Here's how the part is built. I have some questions about the finished solid (model axes, mm). Give positions to 0.01 mm unless a question says otherwise; leave off trailing zeros. Order: outer loops, then holes, each group sorted by start corner. A loop starts at its lowest first (then second) coordinate and runs counter-clockwise, first axis right, second up.
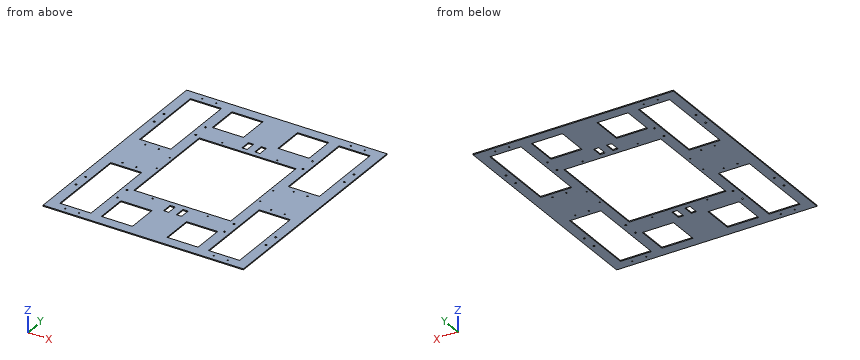
from build123d import *

# Parameters (mm, degrees)
SKETCH_1_W          = 580
SKETCH_1_H          = 660
EXTRUDE_1_DEPTH     = 3
SKETCH_2_W          = 90
SKETCH_2_H          = 233.23
CUT_EXTRUDE_1_DEPTH = 3
SKETCH_3_W          = 90
SKETCH_3_H          = 90
CUT_EXTRUDE_2_DEPTH = 4
SKETCH_4_W          = 280
SKETCH_4_H          = 300
CUT_EXTRUDE_3_DEPTH = 3
SKETCH_5_W          = 15
SKETCH_5_H          = 30
CUT_EXTRUDE_4_DEPTH = 3
SKETCH_6_R          = 2
CUT_EXTRUDE_5_DEPTH = 4
SKETCH_7_R          = 2.75
CUT_EXTRUDE_6_DEPTH = 4
SKETCH_8_R          = 2
CUT_EXTRUDE_7_DEPTH = 3


with BuildPart() as part:
    # 草圖1 → 填料-伸長1 (new body)
    with BuildSketch(Plane.XY):
        with Locations((-114.793886735, -166.775956284)):
            Rectangle(SKETCH_1_W, SKETCH_1_H)
    extrude(amount=EXTRUDE_1_DEPTH)

    # 草圖2 → 除料-伸長1 (cut)
    with BuildSketch(Plane.XY.offset(3)):
        with Locations((-329.793886735, -350.160956284)):
            Rectangle(SKETCH_2_W, SKETCH_2_H)
        with Locations((100.206113265, -350.160956284)):
            Rectangle(SKETCH_2_W, SKETCH_2_H)
        with Locations((100.206113265, 16.609043716)):
            Rectangle(SKETCH_2_W, SKETCH_2_H)
        with Locations((-329.793886735, 16.609043716)):
            Rectangle(SKETCH_2_W, SKETCH_2_H)
    extrude(amount=-CUT_EXTRUDE_1_DEPTH, mode=Mode.SUBTRACT)

    # 草圖3 → 除料-伸長2 (cut, through all)
    with BuildSketch(Plane.XY.offset(3)):
        with Locations((-209.793886735, -421.775956284)):
            Rectangle(SKETCH_3_W, SKETCH_3_H)
        with Locations((-19.793886735, -421.775956284)):
            Rectangle(SKETCH_3_W, SKETCH_3_H)
        with Locations((-19.793886735, 88.224043716)):
            Rectangle(SKETCH_3_W, SKETCH_3_H)
        with Locations((-209.793886735, 88.224043716)):
            Rectangle(SKETCH_3_W, SKETCH_3_H)
    extrude(amount=-CUT_EXTRUDE_2_DEPTH, mode=Mode.SUBTRACT)

    # 草圖4 → 除料-伸長3 (cut)
    with BuildSketch(Plane.XY.offset(3)):
        with Locations((-114.793886735, -166.775956284)):
            Rectangle(SKETCH_4_W, SKETCH_4_H)
    extrude(amount=-CUT_EXTRUDE_3_DEPTH, mode=Mode.SUBTRACT)

    # 草圖5 → 除料-伸長4 (cut)
    with BuildSketch(Plane.XY.offset(3)):
        with Locations((-96.293886735, -346.775956284)):
            Rectangle(SKETCH_5_W, SKETCH_5_H)
        with Locations((-133.293886735, -346.775956284)):
            Rectangle(SKETCH_5_W, SKETCH_5_H)
        with Locations((-133.293886735, 13.224043716)):
            Rectangle(SKETCH_5_W, SKETCH_5_H)
        with Locations((-96.293886735, 13.224043716)):
            Rectangle(SKETCH_5_W, SKETCH_5_H)
    extrude(amount=-CUT_EXTRUDE_4_DEPTH, mode=Mode.SUBTRACT)

    # 草圖6 → 除料-伸長5 (cut, through all)
    with BuildSketch(Plane.XY.offset(3)):
        with Locations((-349.793886735, -218.545956284)):
            Circle(SKETCH_6_R)
        with Locations((-309.793886735, -218.545956284)):
            Circle(SKETCH_6_R)
        with Locations((-309.793886735, -481.775956284)):
            Circle(SKETCH_6_R)
        with Locations((-349.793886735, -481.775956284)):
            Circle(SKETCH_6_R)
        with Locations((80.206113265, -481.775956284)):
            Circle(SKETCH_6_R)
        with Locations((120.206113265, -481.775956284)):
            Circle(SKETCH_6_R)
        with Locations((80.206113265, -218.545956284)):
            Circle(SKETCH_6_R)
        with Locations((120.206113265, -218.545956284)):
            Circle(SKETCH_6_R)
        with Locations((-309.793886735, 148.224043716)):
            Circle(SKETCH_6_R)
        with Locations((-349.793886735, 148.224043716)):
            Circle(SKETCH_6_R)
        with Locations((-309.793886735, -115.005956284)):
            Circle(SKETCH_6_R)
        with Locations((-349.793886735, -115.005956284)):
            Circle(SKETCH_6_R)
        with Locations((80.206113265, -115.005956284)):
            Circle(SKETCH_6_R)
        with Locations((120.206113265, -115.005956284)):
            Circle(SKETCH_6_R)
        with Locations((120.206113265, 148.224043716)):
            Circle(SKETCH_6_R)
        with Locations((80.206113265, 148.224043716)):
            Circle(SKETCH_6_R)
    extrude(amount=-CUT_EXTRUDE_5_DEPTH, mode=Mode.SUBTRACT)

    # 草圖7 → 除料-伸長6 (cut, through all)
    with BuildSketch(Plane.XY.offset(3)):
        with Locations((-389.793886735, -368.775956284)):
            Circle(SKETCH_7_R)
        with Locations((-389.793886735, -324.775956284)):
            Circle(SKETCH_7_R)
        with Locations((-269.793886735, -324.775956284)):
            Circle(SKETCH_7_R)
        with Locations((-269.793886735, -368.775956284)):
            Circle(SKETCH_7_R)
        with Locations((40.206113265, -368.775956284)):
            Circle(SKETCH_7_R)
        with Locations((40.206113265, -324.775956284)):
            Circle(SKETCH_7_R)
        with Locations((160.206113265, -324.775956284)):
            Circle(SKETCH_7_R)
        with Locations((160.206113265, -368.775956284)):
            Circle(SKETCH_7_R)
        with Locations((160.206113265, 35.224043716)):
            Circle(SKETCH_7_R)
        with Locations((160.206113265, -8.775956284)):
            Circle(SKETCH_7_R)
        with Locations((40.206113265, -8.775956284)):
            Circle(SKETCH_7_R)
        with Locations((40.206113265, 35.224043716)):
            Circle(SKETCH_7_R)
        with Locations((-269.793886735, 35.224043716)):
            Circle(SKETCH_7_R)
        with Locations((-269.793886735, -8.775956284)):
            Circle(SKETCH_7_R)
        with Locations((-389.793886735, -8.775956284)):
            Circle(SKETCH_7_R)
        with Locations((-389.793886735, 35.224043716)):
            Circle(SKETCH_7_R)
    extrude(amount=-CUT_EXTRUDE_6_DEPTH, mode=Mode.SUBTRACT)

    # 草圖8 → 除料-伸長7 (cut)
    with BuildSketch(Plane.XY.offset(3)):
        with Locations((-194.793886735, -6.775956284)):
            Circle(SKETCH_8_R)
        with Locations((-34.793886735, -6.775956284)):
            Circle(SKETCH_8_R)
        with Locations((-34.793886735, -326.775956284)):
            Circle(SKETCH_8_R)
        with Locations((-194.793886735, -326.775956284)):
            Circle(SKETCH_8_R)
        with Locations((-264.793886735, -136.775956284)):
            Circle(SKETCH_8_R)
        with Locations((-264.793886735, -196.775956284)):
            Circle(SKETCH_8_R)
        with Locations((35.206113265, -136.775956284)):
            Circle(SKETCH_8_R)
        with Locations((35.206113265, -196.775956284)):
            Circle(SKETCH_8_R)
    extrude(amount=-CUT_EXTRUDE_7_DEPTH, mode=Mode.SUBTRACT)


solid = part.part
Q1. I'm going to push flat-ended pins straight in: P1, Ø9, axis at x = 40.21, y = 35.22, coming from the -Z side; P2, Ø3, axis at x = -309.79, y = -218.55, coming from the -Z side. Where does each tip first touch, or does it pass through?
Filled sheet:
P1: stops at z = 0
P2: passes through
Q2. I need wall thicknesses on L1, parallel to Y at x = -223, z = 1.1; L2, parallel to Y at x = -97.5, z = 1; L3, parallel to X at y = -436.5, z = 2.35. Which ranges of each line are inside material? Lowest first, please.
Filled sheet:
L1: y = -496.78 to -466.78, -376.78 to -316.78, -16.78 to 43.22, 133.22 to 163.22
L2: y = -496.78 to -361.78, -331.78 to -316.78, -16.78 to -1.78, 28.22 to 163.22
L3: x = -404.79 to -374.79, -284.79 to -254.79, -164.79 to -64.79, 25.21 to 55.21, 145.21 to 175.21
Q3. If we section it at B-B on x = -153.5: List the corners of the cut face in (y, z) for me.
Filled sheet:
outline: (-496.78, 0) - (-316.78, 0) - (-316.78, 3) - (-496.78, 3) - close; (-16.78, 0) - (163.22, 0) - (163.22, 3) - (-16.78, 3) - close
Q4. If we section it at D-D on y = -282: List the corners of the cut face in (x, z) for me, plus the area to 3 significant figures.
Filled sheet:
outline: (-404.79, 0) - (-374.79, 0) - (-374.79, 3) - (-404.79, 3) - close; (-284.79, 0) - (-254.79, 0) - (-254.79, 3) - (-284.79, 3) - close; (25.21, 0) - (55.21, 0) - (55.21, 3) - (25.21, 3) - close; (145.21, 0) - (175.21, 0) - (175.21, 3) - (145.21, 3) - close
area: 360 mm2
Q5. If we section it at A-A on y = 55: List the corners of the cut face in (x, z) for me.
Filled sheet:
outline: (-404.79, 0) - (-374.79, 0) - (-374.79, 3) - (-404.79, 3) - close; (-284.79, 0) - (-254.79, 0) - (-254.79, 3) - (-284.79, 3) - close; (-164.79, 0) - (-64.79, 0) - (-64.79, 3) - (-164.79, 3) - close; (25.21, 0) - (55.21, 0) - (55.21, 3) - (25.21, 3) - close; (145.21, 0) - (175.21, 0) - (175.21, 3) - (145.21, 3) - close
Q6. If we section it at C-C on x = -14: List the corners of the cut face in (y, z) for me.
Filled sheet:
outline: (-496.78, 0) - (-466.78, 0) - (-466.78, 3) - (-496.78, 3) - close; (-376.78, 0) - (-316.78, 0) - (-316.78, 3) - (-376.78, 3) - close; (-16.78, 0) - (43.22, 0) - (43.22, 3) - (-16.78, 3) - close; (133.22, 0) - (163.22, 0) - (163.22, 3) - (133.22, 3) - close
